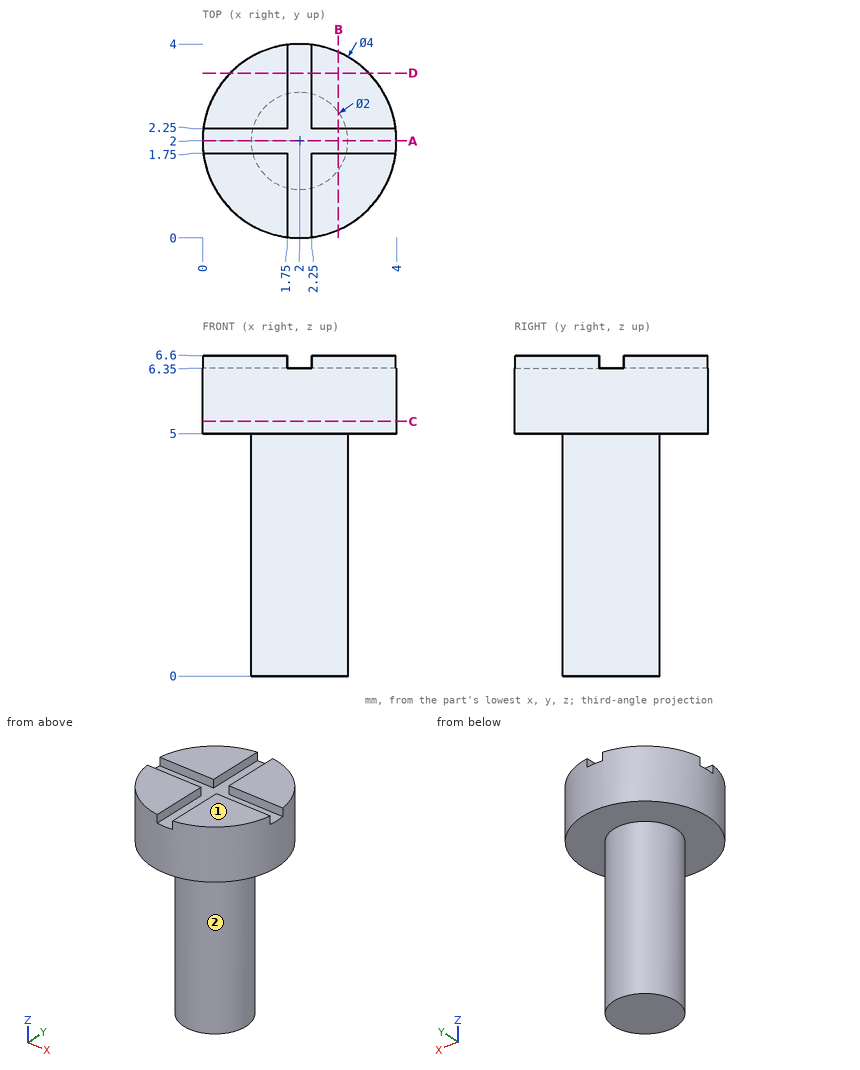
Design review of the part shown in the three views and the two pictorial views. Dimensions are in mm from the part's minimum x, y and z. A direction names the side the tool comes from. Give positions to 0.01 mm unless a question says otherwise; leave off trailing zeros. Loops run counter-clockwise (first coordinate to the right, second up) from the corner with the lowest first, then second, coordinate; pieces in that order, holes last. Notation, with made-up numbers: M -40,-17 L -22,-17 A30 cw -22,12 Z; hole C 72.5,-28.75 d10. An arc over 180 degrees is marked long. Answer as a JSON object with one key per item and string values. Group by question number.
Q1. Add section B-B on x = 2.8. Give the boundary of the cut face in (y, z), and give its area (3 significant figures).
Q2. Tool access review of the marked faces 1 and 2: name each direction out of +Z, -Z, +X, -X, +Y, -Y from which nothing blocks a thin tool from reaching the whole face with its end or side.
Q3. Add section A-A on y = 2. Give the boundary of the cut face in (x, z).
Q4. Insertion check: P1, Ø1, axis at x = 3, z = 3.5, coming from the +Y side; P2, Ø2, axis at y = 0.5, z = 5.5, coming from the +X side; P3, Ø2, axis at y = 1.5, z = 2, coming from the +X side. Each pin has a flat end and moves straight along its axis. Give the tip position at first contact, or say it passes through.
Q5. For probe 1 along Z at (x, y) = (1.85, 3.05); probe 2 along Z at (x, y) = (2.35, 3.45); probe 3 along Y at (x, z) = (1.95, 0.75), list the stretches that pass through material, from the lowest coordinate up. Write a range as [from, to].
Q6. Add section C-C on z = 5.25. Give the boundary of the cut face in (x, y), and give its area (3 significant figures).
Q7. Add section D-D on y = 3.4. Give the boundary of the cut face in (x, z).
Checked values:
{
 "1": {"outline": "M 0.17,5 L 1.4,5 L 1.4,0 L 2.6,0 L 2.6,5 L 3.83,5 L 3.83,6.6 L 2.25,6.6 L 2.25,6.35 L 1.75,6.35 L 1.75,6.6 L 0.17,6.6 Z", "area": "11.7 mm²"},
 "2": {"face 1": "+Z, +X, -X, +Y, -Y", "face 2": "-Z"},
 "3": {"outline": "M 0,5 L 1,5 L 1,0 L 3,0 L 3,5 L 4,5 L 4,6.35 L 0,6.35 Z"},
 "4": {"P1": "y = 2.87", "P2": "x = 3.94", "P3": "x = 3"},
 "5": {"probe 1": "[5, 6.35]", "probe 2": "[5, 6.6]", "probe 3": "[1, 3]"},
 "6": {"outline": "C 2,2 d4", "area": "12.6 mm²"},
 "7": {"outline": "M 0.57,5 L 3.43,5 L 3.43,6.6 L 2.25,6.6 L 2.25,6.35 L 1.75,6.35 L 1.75,6.6 L 0.57,6.6 Z"}
}
